The figure shows three views and two pictorial views of one solid part (mm, origin at its lowest corner). Answer the questions. Give positions to 0.01 mm unless a question says otherwise; leave off trailing zeros. Loops run counter-clockwise (first coordinate to the right, second up) from the corner with the lowest first, then second, coordinate; pieces in that order, holes last. Notation, with made-up numbers: (-9.5, 0) - (-4.5, 0) arc R22 cw to (-4.5, 8) - close; hole circle Ø5 at (10.25, -40). An arc over 180 degrees is marked (long way). Write item = value, one per line.
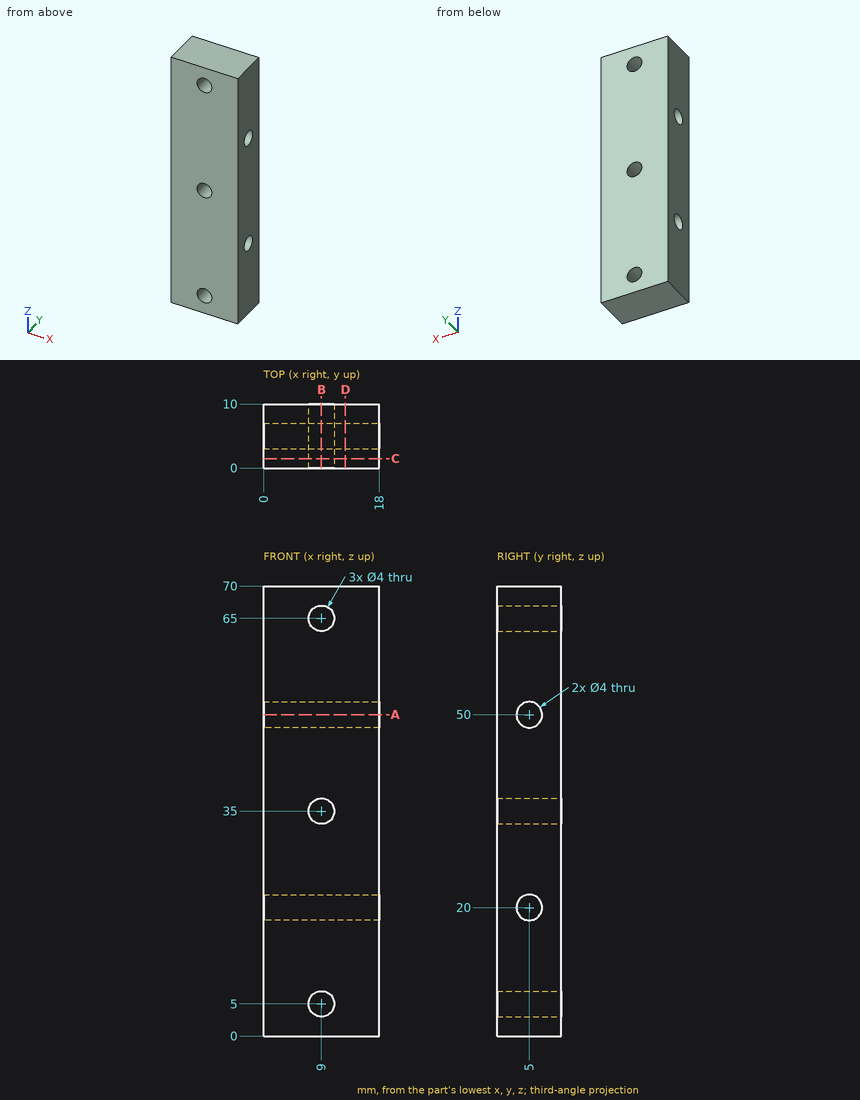
1) A cutting plane is placed at B-B on x = 9. Determine the outline of the cut face in (y, z), then the cut area to 3 significant figures.
Output:
outline = (0, 0) - (10, 0) - (10, 3) - (0, 3) - close; (0, 7) - (10, 7) - (10, 33) - (0, 33) - close; (0, 37) - (10, 37) - (10, 63) - (0, 63) - close; (0, 67) - (10, 67) - (10, 70) - (0, 70) - close; hole circle Ø4 at (5, 20); hole circle Ø4 at (5, 50)
area = 555 mm²
2) A cutting plane is placed at A-A on z = 50. Determine the outline of the cut face in (x, y), then the cut area to 3 significant figures.
Output:
outline = (0, 0) - (18, 0) - (18, 3) - (0, 3) - close; (0, 7) - (18, 7) - (18, 10) - (0, 10) - close
area = 108 mm²
3) A cutting plane is placed at C-C on y = 1.5. Determine the outline of the cut face in (x, z), then the cut area to 3 significant figures.
Output:
outline = (0, 0) - (18, 0) - (18, 70) - (0, 70) - close; hole circle Ø4 at (9, 5); hole circle Ø4 at (9, 35); hole circle Ø4 at (9, 65)
area = 1,220 mm²
4) Find the intervals of material crossed by probe 1 along X at (y, z) = (4.25, 65); probe 2 along Z at (x, y) = (9, 3.5); probe 3 along Z at (x, y) = (10.25, 1.5), in increasing order.
Output:
probe_1 = 0 to 7, 11 to 18
probe_2 = 0 to 3, 7 to 18.68, 21.32 to 33, 37 to 48.68, 51.32 to 63, 67 to 70
probe_3 = 0 to 3.44, 6.56 to 33.44, 36.56 to 63.44, 66.56 to 70
5) A cutting plane is placed at D-D on x = 12.75. Determine the outline of the cut face in (y, z).
Output:
outline = (0, 0) - (10, 0) - (10, 70) - (0, 70) - close; hole circle Ø4 at (5, 20); hole circle Ø4 at (5, 50)
